Geometry check sheet. Reference: the model listing, model coordinates, mm. Face numbers are marked on the shaded views. A direction names the side the tool comes from. Round coordinates to 2 decimals unless told otherwise and drop trailing zeros. Order: outer loops, then holes, each group sorted by start corner. A loop starts at its lowest first (then second) coordinate and runs counter-clockwise, first axis right, second up. Notation, with made-up numbers: (11.5, 76.5) -> (57.5, 76.5) arc R4 ccw to (57.5, 82.5) -> close; hole circle Ø10 at (10.25, 40.5). An arc over 180 degrees is marked (long way). Use a Markdown table: item, result. Add a question column.
Item 1: Sectioned sample at D-D, the plane y = -20.5. Record the cut outline in (x, z), and give its area (3 significant figures).
Item 2: Sectioned sample at C-C, the plane x = 0. Record the cut outline in (y, z).
Item 3: Sectioned sample at A-A, the plane z = -14.7. Record the cut outline in (x, y), and give its area (3 significant figures).
Item 4: Sectioned sample at B-B, the plane z = -7.7. Record the cut outline in (x, y), and give its area (3 significant figures).
Item 5: Set-up check for the marked faces 1 and 2: record each of +Z, -Z, +X, -X, +Y, -Y from which the full face is reachable in a straight line by a thin tool's end or side.
Item 6: Material ranges on probe 1 along X at (y, z) = (2, -21.7); probe 2 along Z at (x, y) = (8, 0.85); probe 3 along Z at (x, y) = (-8, 2.05), recorded low to high. Write a range as [from, to].
Item 7: Gauge pin test, flat ends, axial feed: pin 1 Ø2.5 at (x, y) = (-8.97, -17.8) entering from -Z; pin 2 Ø3.5 at (x, z) = (-8, -7.7) entering from -Y; pin 3 Ø8 at (x, y) = (-5, -17.5) entering from -Z. Record the tip position at first contact, or that the pin passes through.
Item 8: Mould release check, pull along Y, two halves, no side actions. Record for the marked faces 3, 4 and 5: pulls with the +Y half, pulls with the -Y half, needs draft (parallel to the pull), parting line crosses it, or undercut.
Autodesk Inventor part; units mm, degrees
ref_plane "Work Plane1" through (13.1, -2, 0) normal (0, 0, -1) x (-1, 0, 0)
ref_plane "YZ Plane" through (0, 0, 0) normal (1, 0, 0) x (0, 1, 0)
ref_plane "XZ Plane" through (0, 0, 0) normal (0, 1, 0) x (-1, 0, 0)
sketch "Sketch1" plane through (0, 0, 0) normal (1, 0, 0) x (0, 1, 0)
  line L0 (-30.3, 0) -> (0, 0)
  line L1 (0, 0) -> (0, -30)
  line L2 (0, -30) -> (3, -30)
  line L3 (3, -30) -> (3, 3)
  line L4 (3, 3) -> (-30.3, 3)
  line L5 (-30.3, 3) -> (-30.3, 0)
  dimension "d0" = 3
  dimension "d1" = 3
  dimension "d35" = 33.3
  dimension "d36" = 33
extrude "Extrusion1" add sketch "Sketch1" along normal mid plane 26.2
fillet "Fillet2" radius 12.5 2 edges at (-13.1, -30.3, 1.5) (13.1, -30.3, 1.5)
ref_plane "Work Plane1" through (13.1, -2, 0) normal (0, 0, -1) x (-1, 0, 0)
sketch "Sketch2" plane through (13.1, -2, 0) normal (0, 0, -1) x (-1, 0, 0)
  circle A0 centre (22.0664, -15.8) radius 1.5
  circle A1 centre (5.0664, -15.8) radius 1.5
  line L0 (22.0664, -15.8) -> (5.0664, -15.8) construction
  line L1 (5.0664, -15.8) -> (0.9327, -15.8) construction
  circle A2 centre (13.5664, -15.8) radius 4
  line L2 (26.2, 2) -> (26.2, -15.8)
  line L3 (26.2, -15.8) -> (22.0664, -15.8) construction
  point P0 (13.1, 2)
  dimension "d8" = 3
  dimension "d9" = 3
  dimension "d10" = 17
  dimension "d11" = 8
extrude "Extrusion2" cut sketch "Sketch2" against normal through all
sketch "Sketch6" plane through (-13.1, 3, 3) normal (0, 1, 0) x (1, 0, 0)
  line L0 (26.2, 0) -> (0, 0)
  line L1 (26.2, 33) -> (0, 33)
  line L2 (13.1, 33) -> (13.1, 0) construction
  circle A0 centre (13.1, 17.7) radius 5
  line L3 (5.1, 24.7) -> (21.1, 24.7) construction
  line L4 (21.1, 24.7) -> (21.1, 10.7) construction
  line L5 (21.1, 10.7) -> (5.1, 10.7) construction
  line L6 (5.1, 10.7) -> (5.1, 24.7) construction
  line L7 (5.1, 24.7) -> (21.1, 10.7) construction
  line L8 (21.1, 24.7) -> (5.1, 10.7) construction
  circle A1 centre (21.1, 10.7) radius 1.5
  circle A2 centre (5.1, 10.7) radius 1.5
  circle A3 centre (5.1, 24.7) radius 1.5
  circle A4 centre (21.1, 24.7) radius 1.5
  point P0 (13.1, 3)
  dimension "d39" = 10
  dimension "d40" = 17.7
  dimension "d41" = 16
  dimension "d42" = 14
  dimension "d43" = 3
  dimension "d44" = 3
  dimension "d45" = 3
  dimension "d46" = 3
extrude "Extrusion4" cut sketch "Sketch6" against normal up to next
fillet "Fillet3" radius 2 2 edges at (0, 3, 3) (0, 0, 0)
equation "\"d1\" = d0"
properties part number "soporte motor"
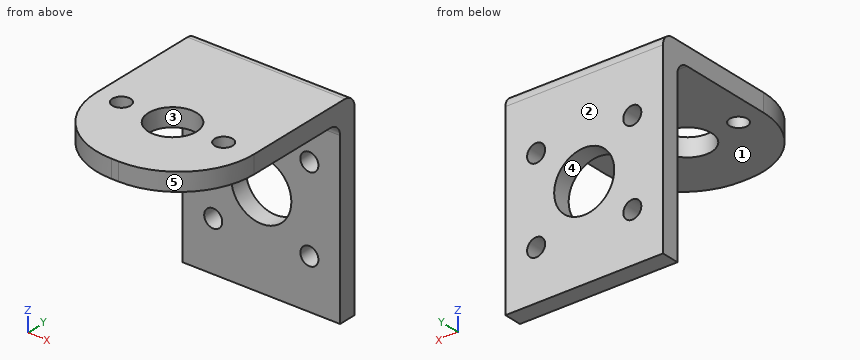
Found:
| question | item | result |
|---|---|---|
| 1 | outline | (-12.8, 0) -> (-3.42, 0) -> (-3.42, 3) -> (-12.8, 3) -> close; (2.48, 0) -> (12.8, 0) -> (12.8, 3) -> (2.48, 3) -> close |
| 1 | area | 59.1 mm2 |
| 2 | outline | (-30.3, 0) -> (-21.77, 0) -> (-21.77, 3) -> (-30.3, 3) -> close; (-13.83, 0) -> (-2, 0) arc R2 cw to (0, -2) -> (0, -9.7) -> (3, -9.7) -> (3, 1) arc R2 ccw to (1, 3) -> (-13.83, 3) -> close; (0, -30) -> (3, -30) -> (3, -19.7) -> (0, -19.7) -> close |
| 3 | outline | (-13.1, 0) -> (-5, 0) -> (-5, 3) -> (-13.1, 3) -> close; (5, 0) -> (13.1, 0) -> (13.1, 3) -> (5, 3) -> close |
| 3 | area | 48.6 mm2 |
| 4 | outline | (-13.1, 0) -> (-9.5, 0) -> (-9.5, 3) -> (-13.1, 3) -> close; (-6.5, 0) -> (6.5, 0) -> (6.5, 3) -> (-6.5, 3) -> close; (9.5, 0) -> (13.1, 0) -> (13.1, 3) -> (9.5, 3) -> close |
| 4 | area | 60.6 mm2 |
| 5 | face 1 | -Z, +X, -X, -Y |
| 5 | face 2 | +Z, -Z, +X, -X, +Y |
| 6 | probe 1 | x = [-13.1, -9.5], [-6.5, 6.5], [9.5, 13.1] |
| 6 | probe 2 | z = [-30, -23.2], [-20.2, -9.2], [-6.2, 3] |
| 6 | probe 3 | z = [-30, -23.2], [-20.2, -9.2], [-6.2, 2.7] |
| 7 | pin 1 | passes through |
| 7 | pin 2 | stops at y = 0 |
| 7 | pin 3 | stops at z = 0 |
| 8 | face 3 | undercut |
| 8 | face 4 | needs draft |
| 8 | face 5 | pulls with the -Y half |
